Verification items for the finished model (mm, model axes). Coordinates: 2 decimals unless noted, no trailing zeros. Write each loop counter-clockwise with the first axis right and the second up, starting at its lowest first coordinate (ties: lowest second). Pieces come first, ordered by that corner, then holes. Notation, with made-up numbers: (62.5, 61.25) - (107.5, 61.25) arc R17 ccw to (107.5, 93.25) - close; hole circle Ø5 at (-26, 54.5). An arc over 180 degrees is marked (long way). Use CSV: the item, a comma, the result in double quotes. Start each with the question number.
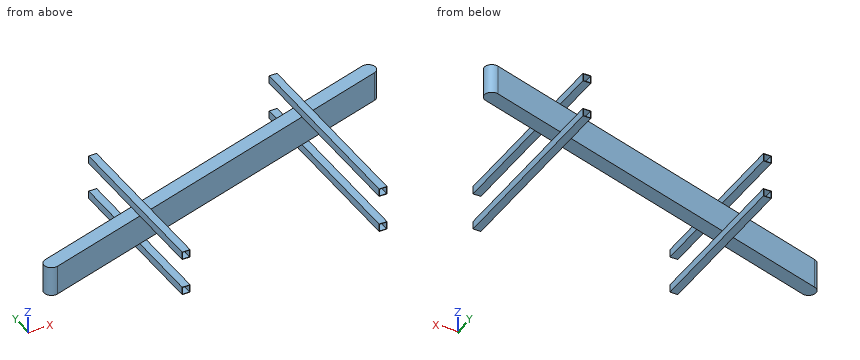
```python
from build123d import *

# Parameters (mm, degrees)
BOSS_EXTRUDE1_DEPTH = 150
SKETCH3_W           = 40
SKETCH3_H           = 40
SKETCH3_W_2         = 36
SKETCH3_H_2         = 36
BOSS_EXTRUDE2_DEPTH = 850
SKETCH4_W           = 40
SKETCH4_H           = 40
SKETCH4_W_2         = 36
SKETCH4_H_2         = 36
BOSS_EXTRUDE3_DEPTH = 1000


with BuildPart() as part:
    # Sketch1 → Boss-Extrude1 (new body)
    with BuildSketch(Plane.XY):
        with BuildLine():
            Line((-11.326300276, 295.748635247), (1942.932426579, 914.919717023))
            ThreePointArc((1942.932426579, 914.919717023), (1990.007362103, 890.497382052), (1965.585027132, 843.422446529))
            Line((1965.585027132, 843.422446529), (11.326300276, 224.251364753))
            ThreePointArc((11.326300276, 224.251364753), (-35.748635247, 248.673699724), (-11.326300276, 295.748635247))
        make_face()
    extrude(amount=BOSS_EXTRUDE1_DEPTH)

    # Sketch3 → Boss-Extrude2 (add)
    with BuildSketch(Plane(origin=(0, 0, 0), x_dir=(1, 0, 0), z_dir=(0, 1, 0))):
        with Locations((538.673699724, 20)):
            Rectangle(SKETCH3_W, SKETCH3_H)
        with Locations((538.673699724, 20)):
            Rectangle(SKETCH3_W_2, SKETCH3_H_2, mode=Mode.SUBTRACT)
        with Locations((538.673699724, -170)):
            Rectangle(SKETCH3_W, SKETCH3_H)
        with Locations((538.673699724, -170)):
            Rectangle(SKETCH3_W_2, SKETCH3_H_2, mode=Mode.SUBTRACT)
    extrude(amount=BOSS_EXTRUDE2_DEPTH)

    # Sketch4 → Boss-Extrude3 (add)
    with BuildSketch(Plane(origin=(0, 0, 0), x_dir=(1, 0, 0), z_dir=(0, 1, 0))):
        with Locations((1538.673699724, 20)):
            Rectangle(SKETCH4_W, SKETCH4_H)
        with Locations((1538.673699724, 20)):
            Rectangle(SKETCH4_W_2, SKETCH4_H_2, mode=Mode.SUBTRACT)
        with Locations((1538.673699724, -170)):
            Rectangle(SKETCH4_W, SKETCH4_H)
        with Locations((1538.673699724, -170)):
            Rectangle(SKETCH4_W_2, SKETCH4_H_2, mode=Mode.SUBTRACT)
    extrude(amount=BOSS_EXTRUDE3_DEPTH)


solid = part.part
```
Q1. Cross-section at D-D (x = 340). Record the cut outline in (y, z), plus the area to 3 significant figures.
Q2. Gauge pin test, flat ends, axial feed: pin 1 (6 mm diameter, centred on x = 1415, z = 148.5, fed in from -Y); pin 2 (1 mm diameter, centred on x = 509.5, z = 67.5, fed in from +Y); pin 3 (20 mm diameter, centred on y = 501, z = 173.5, fed in from -X). Record the tip position at first contact, or that the pin passes through.
Q3. Scan lines: line 1 along X through (y, z) = (157.5, 162); line 2 along Z through (x, y) = (520, 174); line 3 along Y through (x, z) = (635.5, 1.5). Record each from-to range of solid material in increasing order. Write a range as from..to.
Q4. Cross-section at B-B (z = 65). Record the cut outline in (x, y).
Q5. Cross-section at A-A (y = 751.5). State how many separate pieces and enclosed holes the cut face has, plus the area to 3 significant figures.
Reply:
1,outline,"(328.39, 0) - (407.06, 0) - (407.06, 150) - (328.39, 150) - close"
1,area,"11,800 mm^2"
2,pin 1,"y = 668.03"
2,pin 2,"y = 460.92"
2,pin 3,"x = 518.67"
3,line 1,"518.67..520.67, 556.67..558.67, 1518.67..1520.67, 1556.67..1558.67"
3,line 2,"-40..0, 150..190"
3,line 3,"422.01..500.68"
4,outline,"(-11.33, 295.75) arc R37.5 ccw to (11.33, 224.25) - (1965.59, 843.42) arc R37.5 ccw to (1942.93, 914.92) - close"
5,separate pieces,"3"
5,enclosed holes,"4"
5,area,"38,500 mm^2"
